Work out the finished part from the listing and answer in its coordinate system (mm). A direction names the side the tool comes from. Round coordinates to 2 decimals unless told otherwise and drop trailing zeros. Write each loop counter-clockwise with the first axis right and the second up, starting at its lowest first coordinate (ties: lowest second). Pieces come first, ordered by that corner, then holes. Notation, with made-up numbers: (-18.75, -21.5) - (-10.75, -21.5) arc R20 cw to (-10.75, -2.5) - close; hole circle Ø2 at (80, -25.75). An arc over 180 degrees is marked (long way). Answer as a JSON object with one key per item and string values.
Solid Edge part; units mm, degrees
sketch "Sketch1" plane through (0, 0, 0) normal (0, -1, 0) x (1, 0, 0)
  line L0 (40, -27) -> (40, 27)
  line L1 (40, 27) -> (-40, 27)
  line L2 (-40, 27) -> (-40, -27)
  line L3 (-40, -27) -> (40, -27)
extrude "Protrusion1" add sketch "Sketch1" along normal blind 2
sketch "Sketch2" plane through (0, 0, 0) normal (0, -1, 0) x (1, 0, 0)
  line L0 (-25, 23) -> (-15, 23)
  line L1 (-15, 23) -> (-15, 25)
  line L2 (-15, 25) -> (-25, 25)
  line L3 (-25, 25) -> (-25, 23)
extrude "ExtrudedCutout_1" cut sketch "Sketch2" along normal blind 2
sketch "Sketch3" plane through (0, 0, 0) normal (0, -1, 0) x (1, 0, 0)
  line L0 (25, 25) -> (15, 25)
  line L1 (15, 25) -> (15, 23)
  line L2 (15, 23) -> (25, 23)
  line L3 (25, 23) -> (25, 25)
extrude "ExtrudedCutout_2" cut sketch "Sketch3" along normal blind 2
sketch "Sketch4" plane through (0, 0, 0) normal (0, -1, 0) x (1, 0, 0)
  line L0 (15, -25) -> (25, -25)
  line L1 (25, -25) -> (25, -23)
  line L2 (25, -23) -> (15, -23)
  line L3 (15, -23) -> (15, -25)
extrude "ExtrudedCutout_3" cut sketch "Sketch4" along normal blind 2
sketch "Sketch5" plane through (0, 0, 0) normal (0, -1, 0) x (1, 0, 0)
  line L0 (-15, -23) -> (-25, -23)
  line L1 (-25, -23) -> (-25, -25)
  line L2 (-25, -25) -> (-15, -25)
  line L3 (-15, -25) -> (-15, -23)
extrude "ExtrudedCutout_4" cut sketch "Sketch5" along normal blind 2
sketch "Sketch6" plane through (0, 0, 0) normal (0, -1, 0) x (1, 0, 0)
  line L0 (-38, -27) -> (-38, -5)
  line L1 (-38, -5) -> (-40, -5)
  line L2 (-40, -5) -> (-40, -27)
  line L3 (-40, -27) -> (-38, -27)
extrude "ExtrudedCutout_5" cut sketch "Sketch6" along normal blind 2
sketch "Sketch7" plane through (0, 0, 0) normal (0, -1, 0) x (1, 0, 0)
  line L0 (-38, 5) -> (-38, 27)
  line L1 (-38, 27) -> (-40, 27)
  line L2 (-40, 27) -> (-40, 5)
  line L3 (-40, 5) -> (-38, 5)
extrude "ExtrudedCutout_6" cut sketch "Sketch7" along normal blind 2
sketch "Sketch8" plane through (0, 0, 0) normal (0, -1, 0) x (1, 0, 0)
  line L0 (38, -5) -> (38, -27)
  line L1 (38, -27) -> (40, -27)
  line L2 (40, -27) -> (40, -5)
  line L3 (40, -5) -> (38, -5)
extrude "ExtrudedCutout_7" cut sketch "Sketch8" along normal blind 2
sketch "Sketch9" plane through (0, 0, 0) normal (0, -1, 0) x (1, 0, 0)
  line L0 (38, 27) -> (38, 5)
  line L1 (38, 5) -> (40, 5)
  line L2 (40, 5) -> (40, 27)
  line L3 (40, 27) -> (38, 27)
extrude "ExtrudedCutout_8" cut sketch "Sketch9" along normal blind 2
sketch "Sketch10" plane through (0, 0, 0) normal (0, -1, 0) x (1, 0, 0)
  line L0 (-19.25, -2) -> (-9, -2)
  line L1 (-9, -2) -> (-9, 9)
  line L2 (-9, 9) -> (-19.25, 9)
  line L3 (-19.25, 9) -> (-19.25, -2)
extrude "ExtrudedCutout_9" cut sketch "Sketch10" along normal blind 2
properties material "Acrylic, high impact grade"
Item 1: A cutting plane is placed at B-B (x = -10). Write down the section's boundary in (y, z).
Results found:
{"outline": "(-2, -27) - (0, -27) - (0, -2) - (-2, -2) - close; (-2, 9) - (0, 9) - (0, 27) - (-2, 27) - close"}
Item 2: A cutting plane is placed at D-D (x = 16.5). Write down the section's boundary in (y, z).
Results found:
{"outline": "(-2, -27) - (0, -27) - (0, -25) - (-2, -25) - close; (-2, -23) - (0, -23) - (0, 23) - (-2, 23) - close; (-2, 25) - (0, 25) - (0, 27) - (-2, 27) - close"}
Item 3: Consider line 1 along Z through (x, y) = (20.5, -1.55); line 2 along X through (y, z) = (-0.1, 2); line 3 along X through (y, z) = (-0.65, 6). Determine where each line is inside the solid, lowest interval first.
Results found:
{"line 1": "-27 to -25, -23 to 23, 25 to 27", "line 2": "-40 to -19.25, -9 to 40", "line 3": "-38 to -19.25, -9 to 38"}
Item 4: A cutting plane is placed at A-A (z = 6). Write down the section's boundary in (x, y).
Results found:
{"outline": "(-38, -2) - (-19.25, -2) - (-19.25, 0) - (-38, 0) - close; (-9, -2) - (38, -2) - (38, 0) - (-9, 0) - close"}
Item 5: Each of these flat-tipped pins is pushed along its axis until it touches: P1, Ø0.6, axis at x = -39.5, y = -1.5, coming from the -Z side; P2, Ø1, axis at y = -0.5, z = -11.5, coming from the -X side; P3, Ø0.6, axis at y = -1, z = 23.5, coming from the +X side. Where does it stop, or does it pass through?
Results found:
{"P1": "z = -5", "P2": "x = -38", "P3": "x = 38"}
Item 6: A cutting plane is placed at C-C (y = -1.35). Give the number of separate pieces and of enclosed holes in the cut face, and give its area (3 significant figures).
Results found:
{"separate pieces": "1", "enclosed holes": "5", "area": "3,950 mm²"}
Item 7: For faces 1 (the flat face through (38, -1, 16)), 2 (the flat face through (-38, -1, -16)), 3 (the flat face through (20, -1, -25)), 4 (the flat face through (-38, -1, 16)), determine the directions among +Z, -Z, +X, -X, +Y, -Y from which every point of the face is accessible in a straight line to the end or side of a thin tool.
Results found:
{"face 1": "+Z, +X, +Y, -Y", "face 2": "-Z, -X, +Y, -Y", "face 3": "+Y, -Y", "face 4": "+Z, -X, +Y, -Y"}
Item 8: Determine the mould class of faces 5 (the flat face through (1, 0, 0)), 6 (the flat face through (25, -1, 24)), 7 (the flat face through (1, -1, 27)) for opening direction Z: pulls with the +Z half, pulls with the -Z half, needs draft (parallel to the pull), parting line crosses it, or undercut.
Results found:
{"face 5": "needs draft", "face 6": "undercut", "face 7": "pulls with the +Z half"}
